```python
from build123d import *

# Parameters (mm, degrees)
F0_R      = 1.55
F0_W      = 3.9
F0_H      = 10
F0_W_2    = 20.36
F0_H_2    = 9
F0_W_3    = 7.4
F0_H_3    = 6.6
F0_R_2    = 3.125
F1_DEPTH  = 1.6
F2_DEPTH  = 8.81
F3_DEPTH  = 3.2
F4_DEPTH  = 1.5
F5_DEPTH  = 5.3
F6_R      = 3.125
F7_DEPTH  = 1.87
F8_R      = 5.88
F9_DEPTH  = 10
F10_W     = 13.8
F10_H     = 12
F11_DEPTH = 5.6
F12_R     = 3.4
F13_DEPTH = 8.4
F14_R     = 7.5
F14_R_2   = 3.4
F15_DEPTH = 3
F16_R     = 5.8
F17_DEPTH = 12.45
F10_W_2   = 6
F10_H_2   = 6
F10_R     = 1.75
F18_DEPTH = 3.5
F19_R     = 1.75
F20_DEPTH = 1.85
F22_W     = 40.3
F22_H     = 1.5
F23_DEPTH = 5.9
F22_W_2   = 98.17
F22_H_2   = 59.93
F22_R     = 1.8
F24_DEPTH = 1.6
F25_W     = 41
F25_H     = 1.7
F26_DEPTH = 4.4
F25_W_2   = 97
F25_H_2   = 40
F27_DEPTH = 9.5


with BuildPart() as f1:
    # F0 (on Top) → F1 (new body)
    with BuildSketch(Plane.XY):
        Polygon((0, 55), (0, 0), (150, 0), (150, 8), (122, 8), (122, 33), (128, 33), (131, 35), (150, 35), (150, 55), align=None)
        with Locations((2.75, 2.75)):
            Circle(F0_R, mode=Mode.SUBTRACT)
        with Locations((147.25, 2.75)):
            Circle(F0_R, mode=Mode.SUBTRACT)
        with Locations((108.65, 16)):
            Rectangle(F0_W, F0_H, mode=Mode.SUBTRACT)
        with Locations((70.18, 28.5)):
            Rectangle(F0_W_2, F0_H_2, mode=Mode.SUBTRACT)
        with Locations((2.75, 52.25)):
            Circle(F0_R, mode=Mode.SUBTRACT)
        with Locations((92.82, 28.5)):
            Rectangle(F0_W_2, F0_H_2, mode=Mode.SUBTRACT)
        with Locations((136.8, 44.2)):
            Rectangle(F0_W_3, F0_H_3, mode=Mode.SUBTRACT)
        with Locations((147.25, 52.25)):
            Circle(F0_R, mode=Mode.SUBTRACT)
        Polygon((122, 8), (150, 8), (150, 35), (131, 35), (128, 33), (122, 33), align=None)
        with Locations((70.18, 28.5)):
            Rectangle(F0_W_2, F0_H_2)
        with Locations((108.65, 16)):
            Rectangle(F0_W, F0_H)
        with Locations((136.8, 44.2)):
            Rectangle(F0_W_3, F0_H_3)
        with Locations((136.8, 44.2)):
            Circle(F0_R_2, mode=Mode.SUBTRACT)
        with Locations((136.8, 44.2)):
            Circle(F0_R_2)
        with Locations((92.82, 28.5)):
            Rectangle(F0_W_2, F0_H_2)
    extrude(amount=-F1_DEPTH)

    # F0 (on Top) → F2 (join)
    with BuildSketch(Plane.XY):
        with Locations((70.18, 28.5)):
            Rectangle(F0_W_2, F0_H_2)
        with Locations((92.82, 28.5)):
            Rectangle(F0_W_2, F0_H_2)
    extrude(amount=F2_DEPTH)

    # F0 (on Top) → F3 (join)
    with BuildSketch(Plane.XY):
        Polygon((122, 8), (150, 8), (150, 35), (131, 35), (128, 33), (122, 33), align=None)
    extrude(amount=F3_DEPTH)

    # F0 (on Top) → F4 (join)
    with BuildSketch(Plane.XY):
        with Locations((108.65, 16)):
            Rectangle(F0_W, F0_H)
    extrude(amount=F4_DEPTH)

    # F0 (on Top) → F5 (join)
    with BuildSketch(Plane.XY):
        with Locations((136.8, 44.2)):
            Rectangle(F0_W_3, F0_H_3)
        with Locations((136.8, 44.2)):
            Circle(F0_R_2, mode=Mode.SUBTRACT)
        with Locations((136.8, 44.2)):
            Circle(F0_R_2)
    extrude(amount=F5_DEPTH)

    # F6 (on face) → F7 (join)
    with BuildSketch(Plane.XY.offset(5.3)):
        with Locations((136.8, 44.2)):
            Circle(F6_R)
    extrude(amount=F7_DEPTH)

    # F8 (on face) → F9 (join)
    with BuildSketch(Plane(origin=(0, 0, -1.6), x_dir=(1, 0, 0), z_dir=(0, 0, -1))):
        with Locations((13.68, -44.82)):
            Circle(F8_R)
    extrude(amount=F9_DEPTH)

    # F10 (on face) → F11 (join)
    with BuildSketch(Plane(origin=(0, 0, -1.6), x_dir=(1, 0, 0), z_dir=(0, 0, -1))):
        with Locations((12.9, -24.7)):
            Rectangle(F10_W, F10_H)
    extrude(amount=F11_DEPTH)

    # F12 (on face) → F13 (join)
    with BuildSketch(Plane(origin=(0, 0, -7.2), x_dir=(1, 0, 0), z_dir=(0, 0, -1))):
        with Locations((12.9, -24.7)):
            Circle(F12_R)
    extrude(amount=F13_DEPTH)

    # F14 (on face) → F15 (join)
    with BuildSketch(Plane(origin=(0, 0, -15.6), x_dir=(1, 0, 0), z_dir=(0, 0, -1))):
        with Locations((12.9, -24.7)):
            Circle(F14_R)
        with Locations((12.9, -24.7)):
            Circle(F14_R_2, mode=Mode.SUBTRACT)
        with Locations((12.9, -24.7)):
            Circle(F14_R_2)
    extrude(amount=F15_DEPTH)

    # F16 (on face) → F17 (join)
    with BuildSketch(Plane(origin=(0, 0, -18.6), x_dir=(1, 0, 0), z_dir=(0, 0, -1))):
        with Locations((12.9, -24.7)):
            Circle(F16_R)
    extrude(amount=F17_DEPTH)

    # F10 (on face) → F18 (join)
    with BuildSketch(Plane(origin=(0, 0, -1.6), x_dir=(1, 0, 0), z_dir=(0, 0, -1))):
        with Locations((13, -8)):
            Rectangle(F10_W_2, F10_H_2)
        with Locations((13, -8)):
            Circle(F10_R, mode=Mode.SUBTRACT)
        with Locations((13, -8)):
            Circle(F10_R)
    extrude(amount=F18_DEPTH)

    # F19 (on face) → F20 (join)
    with BuildSketch(Plane(origin=(0, 0, -5.1), x_dir=(1, 0, 0), z_dir=(0, 0, -1))):
        with Locations((13, -8)):
            Circle(F19_R)
    extrude(amount=F20_DEPTH)

    # F22 (on offset) → F23 (join, through all)
    with BuildSketch(Plane(origin=(0, 0, -7.5), x_dir=(1, 0, 0), z_dir=(0, 0, -1))):
        with Locations((66.28, -50.28)):
            Rectangle(F22_W, F22_H)
    extrude(amount=-F23_DEPTH)

    # F22 (on offset) → F24 (join)
    with BuildSketch(Plane(origin=(0, 0, -7.5), x_dir=(1, 0, 0), z_dir=(0, 0, -1))):
        with Locations((87.415, -22.065)):
            Rectangle(F22_W_2, F22_H_2)
        with Locations((40.82, -49.59)):
            Circle(F22_R, mode=Mode.SUBTRACT)
        with Locations((66.28, -50.28)):
            Rectangle(F22_W, F22_H, mode=Mode.SUBTRACT)
        with Locations((133.7, -49.59)):
            Circle(F22_R, mode=Mode.SUBTRACT)
        with Locations((40.82, 5.3)):
            Circle(F22_R, mode=Mode.SUBTRACT)
        with Locations((133.7, 5.3)):
            Circle(F22_R, mode=Mode.SUBTRACT)
    extrude(amount=-F24_DEPTH)

    # F25 (on face) → F26 (join)
    with BuildSketch(Plane(origin=(0, 0, -7.5), x_dir=(1, 0, 0), z_dir=(0, 0, -1))):
        with Locations((106.7, -51.18)):
            Rectangle(F25_W, F25_H)
    extrude(amount=F26_DEPTH)

    # F25 (on face) → F27 (join)
    with BuildSketch(Plane(origin=(0, 0, -7.5), x_dir=(1, 0, 0), z_dir=(0, 0, -1))):
        with Locations((87.415, -22.1)):
            Rectangle(F25_W_2, F25_H_2)
    extrude(amount=F27_DEPTH)


solid = f1.part
```
Geometry: final body of the model. Coordinates: model frame, mm. A direction names the side the tool comes from. Round coordinates to 2 decimals unless told otherwise and drop trailing zeros. Write each loop counter-clockwise with the first axis right and the second up, starting at its lowest first coordinate (ties: lowest second). Pieces come first, ordered by that corner, then holes. Notation, with made-up numbers: M -25,69 L 19,69 A25 ccw 19,87 Z; hole C 37.25,12 d6. An arc over 180 degrees is marked long. Answer in a Markdown table with one row per item. Add a question column.
(1) Ray query, L1, parallel to Y at x = 133.7, z = -6.35; L2, parallel to X at y = 52, z = -1; L3, parallel to Y at x = 147.25, z = -0.65. Return the intervals inside material, ascending.
(2) Contact query for flat-ended pins moving along their axis: pin 1 (1.7 mm diameter, centred on y = 26, z = -3.5, fed in from -X); pin 2 (7.5 mm diameter, centred on x = 11, y = 22, fed in from +Z); pin 3 (12 mm diameter, centred on y = -0.5, z = -7, fed in from -X); pin 4 (2 mm diameter, centred on y = 16.5, z = -26, fed in from -X). Output: stop coordinate, or through.
(3) Cut plane B-B, the plane y = 13. Return the cut outline in (x, z) (3 decimals), then the cut area to 3 significant figures.
(4) Cut plane C-C, the plane x = 2.75. Return the cut outline in (y, z).
(5) Cut plane A-A, the plane x = 120.5. Return the cut outline in (y, z), then the cut area to 3 significant figures.
(6) Draft query along Y for faces 6 (the face through (136, 22, 3.2)), 7 (the face through (137, 40.9, 3)), 8 (the face through (98, 52.03, -8)). Return one class per face: pulls with the +Y half, pulls with the -Y half, needs draft (parallel to the pull), parting line crosses it, or undercut.
(7) Reachability of faces 1 (the face through (10, 22, -7.2)), 2 (the face through (10, 8, -3)), 3 (the face through (141, 35, 2)), 4 (the face through (87, 42.1, -12)), 5 (the face through (19.288, 43.054, -6.53)) from +Z, -Z, +X, -X, +Y, -Y: full face, straight path, thin tool, end or side. Return the list, or none.
(8) Cut plane D-D, the plane z = -14. Return the cut outline in (x, y) (3 decimals), then the cut area to 3 significant figures.
Established:
| question | item | result |
|---|---|---|
| 1 | L1 | -7.9 to -7.1, -3.5 to 47.79, 51.39 to 52.03 |
| 1 | L2 | 0 to 1.22, 4.28 to 145.72, 148.78 to 150 |
| 1 | L3 | 0 to 1.2, 4.3 to 50.7, 53.8 to 55 |
| 2 | pin 1 | x = 6 |
| 2 | pin 2 | z = 0 |
| 2 | pin 3 | x = 0 |
| 2 | pin 4 | through |
| 3 | outline | M 0,-1.6 L 150,-1.6 L 150,3.2 L 122,3.2 L 122,0 L 110.6,0 L 110.6,1.5 L 106.7,1.5 L 106.7,0 L 0,0 Z; M 38.33,-7.5 L 38.915,-7.5 L 38.915,-17 L 135.915,-17 L 135.915,-7.5 L 136.5,-7.5 L 136.5,-5.9 L 38.33,-5.9 Z |
| 3 | area | 1,410 mm² |
| 4 | outline | M 0,-1.6 L 1.2,-1.6 L 1.2,0 L 0,0 Z; M 4.3,-1.6 L 50.7,-1.6 L 50.7,0 L 4.3,0 Z; M 53.8,-1.6 L 55,-1.6 L 55,0 L 53.8,0 Z |
| 5 | outline | M -7.9,-7.5 L 2.1,-7.5 L 2.1,-17 L 42.1,-17 L 42.1,-7.5 L 50.33,-7.5 L 50.33,-11.9 L 52.03,-11.9 L 52.03,-5.9 L -7.9,-5.9 Z; M 0,-1.6 L 55,-1.6 L 55,0 L 0,0 Z |
| 5 | area | 571 mm² |
| 6 | face 6 | needs draft |
| 6 | face 7 | undercut |
| 6 | face 8 | pulls with the +Y half |
| 7 | face 1 | none |
| 7 | face 2 | -Z, -X, -Y |
| 7 | face 3 | +Z, +X, -X |
| 7 | face 4 | -Z, +X |
| 7 | face 5 | -Z |
| 8 | outline | C 12.9,24.7 d6.8; M 38.915,2.1 L 135.915,2.1 L 135.915,42.1 L 38.915,42.1 Z |
| 8 | area | 3,920 mm² |
